The figure shows three views and two pictorial views of one solid part (mm, origin at its lowest corner). Answer the questions. Give positions to 0.01 mm unless a question says otherwise; leave off trailing zeros. Loops run counter-clockwise (first coordinate to the right, second up) from the corner with the lowest first, then second, coordinate; pieces in that order, holes last. Notation, with made-up numbers: (-37, 44) - (-17, 44) arc R29 cw to (-17, 76) - close; hole circle Ø7 at (35, 59.5). An arc over 180 degrees is marked (long way). Write each question's results on one line, items separated by ' | '.
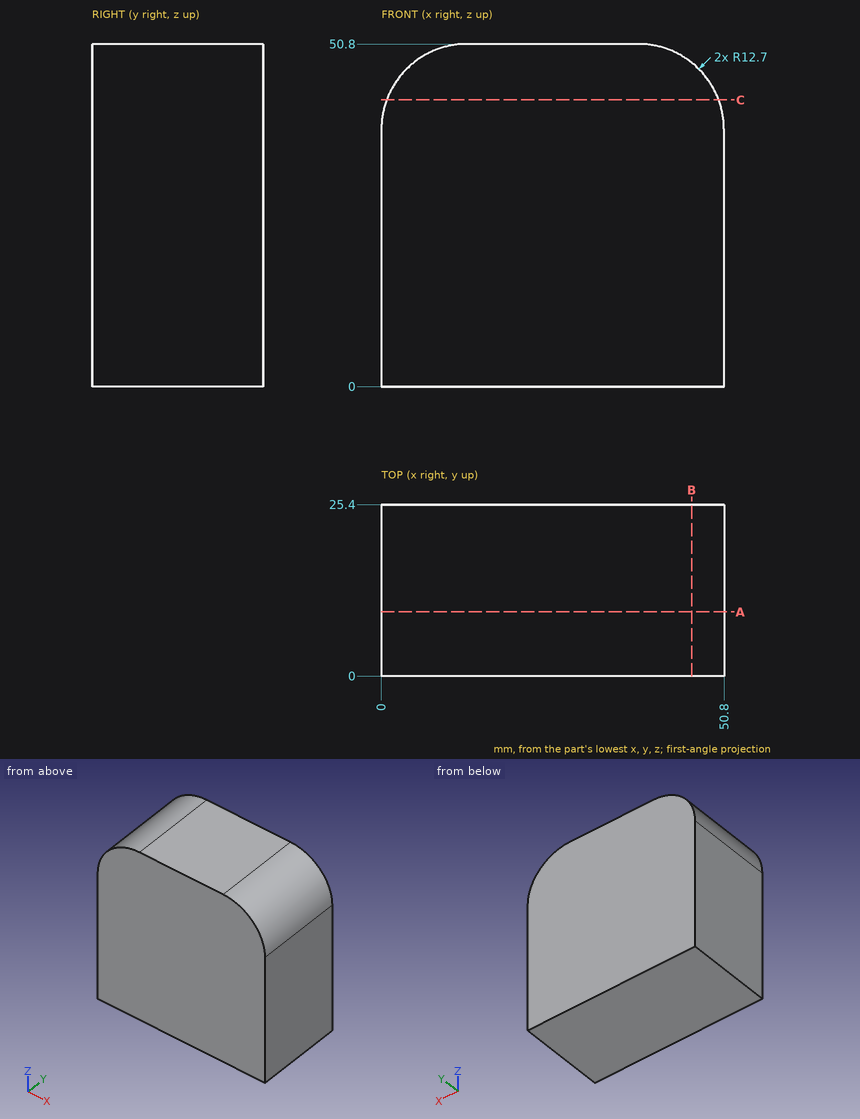
Item 1: A cutting plane is placed at B-B, the plane x = 46. Determine the outline of the cut face in (y, z).
Values found:
outline: (0, 0) - (25.4, 0) - (25.4, 48.04) - (0, 48.04) - close
Item 2: Find the intervals of material crossed by line 1 along Z through (x, y) = (44.5, 21); line 2 along Z through (x, y) = (7.5, 21); line 3 along X through (y, z) = (8.5, 44), in increasing order. Write a range as [from, to].
Values found:
line 1: z = [0, 49.07] | line 2: z = [0, 49.69] | line 3: x = [1.45, 49.35]
Item 3: A cutting plane is placed at C-C, the plane z = 42.5. Determine the outline of the cut face in (x, y), plus the area to 3 significant figures.
Values found:
outline: (0.79, 0) - (50.01, 0) - (50.01, 25.4) - (0.79, 25.4) - close | area: 1,250 mm²
Item 4: Flat-ended cylindrical pins translate along their axes: P1, Ø1.5, axis at x = 45, z = 33, coming from the -Y side; P2, Ø1, axis at y = 19, z = 44.5, coming from the -X side. Find the tip coordinate at first contact, or state that the pin passes through.
Values found:
P1: stops at y = 0 | P2: stops at x = 1.45
Item 5: A cutting plane is placed at A-A, the plane y = 9.5. Determine the outline of the cut face in (x, z).
Values found:
outline: (0, 0) - (50.8, 0) - (50.8, 38.1) arc R12.7 ccw to (38.1, 50.8) - (12.7, 50.8) arc R12.7 ccw to (0, 38.1) - close
